from build123d import *

# Parameters (mm, degrees)
F0_W           = 685.8
F0_H           = 1397
F1_DEPTH       = 711.2
F2_W           = 609.6
F2_H           = 508
F2_H_2         = 88.9
F3_DEPTH       = 800.1
F4_W           = 609.6
F4_H           = 88.9
F5_DEPTH       = 596.901
F6_W           = 609.6
F6_H           = 762
F7_DEPTH       = 9.525
F8_W           = 584.2
F8_H           = 736.6
F9_DEPTH       = 50.8
F10_W          = 609.6
F10_H          = 38.1
F11_DEPTH      = 1397.001
F12_W          = 762
F12_H          = 508
F12_W_2        = 1320.8
F12_H_2        = 127
F13_DEPTH      = 685.801
F14_W          = 609.6
F14_H          = 508
F15_DEPTH      = 584.2
F16_W          = 609.6
F16_H          = 520.7
F17_DEPTH      = 9.525
F18_W          = 584.2
F18_H          = 495.3
F19_DEPTH      = 28.575
F21_DEPTH      = 685.801
F22_W          = 558.8
F22_H          = 38.1
F23_DEPTH      = 558.8
F24_W          = 558.7746
F24_H          = 558.8
F24_R          = 228.6
F25_DEPTH      = 50.8
F26_W          = 38.1
F26_H          = 25.4
F27_DEPTH      = 52.5951328439
F28_W          = 38.1
F28_H          = 38.1
F29_DEPTH      = 127
F29_DEPTH_BACK = 88.9
F30_W          = 609.6
F30_H          = 508
F31_DEPTH      = 12.7
F32_W          = 609.6
F32_H          = 762
F33_DEPTH      = 165.101
F34_W          = 38.1
F34_H          = 38.1
F35_DEPTH      = 762


# Not quite as in the source:
# - a length typed as a fraction of an inch, garbled in the dataset ("3 / 203.2 mm" for 3/8 in), is restored


with BuildPart() as f1:
    # F0 (on Top) → F1 (new body)
    with BuildSketch(Plane.XY):
        Rectangle(F0_W, F0_H)
    extrude(amount=F1_DEPTH)

    # F2 (on face) → F3 (cut)
    with BuildSketch(Plane.XZ.offset(698.5)):
        with Locations((0, 419.1)):
            Rectangle(F2_W, F2_H)
        with Locations((0, 82.55)):
            Rectangle(F2_W, F2_H_2)
    extrude(amount=-F3_DEPTH, mode=Mode.SUBTRACT)

    # F4 (on face) → F5 (cut, through all)
    with BuildSketch(Plane.XZ.offset(-101.6)):
        with Locations((0, 82.55)):
            Rectangle(F4_W, F4_H)
    extrude(amount=-F5_DEPTH, mode=Mode.SUBTRACT)

    # F6 (on face) → F7 (cut)
    with BuildSketch(Plane.XY.offset(711.2)):
        with Locations((0, -279.4)):
            Rectangle(F6_W, F6_H)
    extrude(amount=-F7_DEPTH, mode=Mode.SUBTRACT)

    # F8 (on face) → F9 (cut)
    with BuildSketch(Plane.XY.offset(701.675)):
        with Locations((0, -279.4)):
            Rectangle(F8_W, F8_H)
    extrude(amount=-F9_DEPTH, mode=Mode.SUBTRACT)

    # F10 (on face) → F11 (cut, through all)
    with BuildSketch(Plane.XZ.offset(698.5)):
        with Locations((0, 19.05)):
            Rectangle(F10_W, F10_H)
    extrude(amount=-F11_DEPTH, mode=Mode.SUBTRACT)

    # F12 (on face) → F13 (cut, through all)
    with BuildSketch(Plane(origin=(-342.9, 0, 0), x_dir=(0, -1, 0), z_dir=(-1, 0, 0))):
        with Locations((279.4, 419.1)):
            Rectangle(F12_W, F12_H)
        with Locations((0, 63.5)):
            Rectangle(F12_W_2, F12_H_2)
    extrude(amount=-F13_DEPTH, mode=Mode.SUBTRACT)

    # F14 (on face) → F15 (cut)
    with BuildSketch(Plane(origin=(0, 698.5, 0), x_dir=(-1, 0, 0), z_dir=(0, 1, 0))):
        with Locations((0, 419.1)):
            Rectangle(F14_W, F14_H)
    extrude(amount=-F15_DEPTH, mode=Mode.SUBTRACT)

    # F16 (on face) → F17 (cut)
    with BuildSketch(Plane.XY.offset(711.2)):
        with Locations((0, 400.05)):
            Rectangle(F16_W, F16_H)
    extrude(amount=-F17_DEPTH, mode=Mode.SUBTRACT)

    # F18 (on face) → F19 (cut, through all)
    with BuildSketch(Plane.XY.offset(701.675)):
        with Locations((0, 400.05)):
            Rectangle(F18_W, F18_H)
    extrude(amount=-F19_DEPTH, mode=Mode.SUBTRACT)

    # F20 (on face) → F21 (cut, through all)
    with BuildSketch(Plane.YZ.offset(342.9)):
        Polygon((660.4, 673.1), (647.7, 673.1), (152.4, 673.1), (139.7, 673.1), (139.7, 165.1), (660.4, 165.1), align=None)
    extrude(amount=-F21_DEPTH, mode=Mode.SUBTRACT)

    # F22 (on face) → F23 (join)
    with BuildSketch(Plane.YZ.offset(342.9)):
        with Locations((381, 146.05)):
            Rectangle(F22_W, F22_H)
    extrude(amount=F23_DEPTH)

    # F24 (on face) → F25 (join)
    with BuildSketch(Plane.XY.offset(165.1)):
        with Locations((622.3127, 381)):
            Rectangle(F24_W, F24_H)
        with Locations((622.3, 381)):
            Circle(F24_R, mode=Mode.SUBTRACT)
    extrude(amount=F25_DEPTH)

    # F26 (on face) → F27 (cut, up to face)
    with BuildSketch(Plane.XZ.offset(-101.6)):
        with Locations((622.3, 203.2)):
            Rectangle(F26_W, F26_H)
    extrude(amount=-F27_DEPTH, mode=Mode.SUBTRACT)

    # F28 (on face) → F29 (join, two sides)
    with BuildSketch(Plane(origin=(0, 0, 127), x_dir=(1, 0, 0), z_dir=(0, 0, -1))) as f29_sk:
        with Locations((882.65, -82.55)):
            Rectangle(F28_W, F28_H)
        with Locations((882.65, -679.45)):
            Rectangle(F28_W, F28_H)
        with Locations((361.9619884968, -82.55)):
            Rectangle(F28_W, F28_H)
    extrude(amount=F29_DEPTH)
    extrude(f29_sk.sketch, amount=-F29_DEPTH_BACK)

    # F30 (on face) → F31 (cut, through all)
    with BuildSketch(Plane(origin=(0, 114.3, 0), x_dir=(-1, 0, 0), z_dir=(0, 1, 0))):
        with Locations((0, 419.1)):
            Rectangle(F30_W, F30_H)
    extrude(amount=-F31_DEPTH, mode=Mode.SUBTRACT)

    # F32 (on face) → F33 (cut, through all)
    with BuildSketch(Plane.XY.offset(165.1)):
        with Locations((0, -279.4)):
            Rectangle(F32_W, F32_H)
    extrude(amount=-F33_DEPTH, mode=Mode.SUBTRACT)

    # F34 (on face) → F35 (join, through all)
    with BuildSketch(Plane.XZ.offset(-101.6)):
        with Locations((107.95, 146.05)):
            Rectangle(F34_W, F34_H)
        with Locations((-107.95, 146.05)):
            Rectangle(F34_W, F34_H)
    extrude(amount=F35_DEPTH)


solid = f1.part
Design review of the part built by this model. Coordinates are the model's own, in mm. A direction names the side the tool comes from. Give positions to 0.01 mm unless a question says otherwise; leave off trailing zeros. Write each loop counter-clockwise with the first axis right and the second up, starting at its lowest first coordinate (ties: lowest second). Pieces come first, ordered by that corner, then holes. Notation, with made-up numbers: M 75.5,44 L 89.5,44 A17 cw 89.5,58 Z; hole C 24.25,15.5 d9. An arc over 180 degrees is marked long. Return JSON: item names as keys, results as strings. Group by question number.
Item 1: Clearance check with flat-ended pins moving along their axes: pin 1 Ø8 at (x, y) = (128, -185) entering from +Z; pin 2 Ø11.5 at (x, y) = (628.5, 123.5) entering from +Z; pin 3 Ø2 at (x, y) = (454, 535) entering from +Z. State where each tip first meets the part, or that it passes through.
Item 2: Wall thickness on line 1 along X through (y, z) = (381, 197); line 2 along Y through (x, z) = (321, 254); line 3 along Y through (x, z) = (622.3, 183): over which ranges is each line inside the solid? List them lowest first.
Item 3: Take a section at A-A (x = 202). Give the boundary of the cut face in (y, z) (3 decimals), plus the area to 3 significant figures.
Item 4: Tool access review of faces 3 (the cylindrical face through (727.8, 178.2, 190.1)), 4 (the flat face through (-304.8, 121, 416)), 5 (the flat face through (-304.8, -680, 63)), 6 (the flat face through (882, 660.4, 64)), 7 (the flat face through (2, 107, 673.1)): name each direction out of +Z, -Z, +X, -X, +Y, -Y from which nothing blocks a thin tool from reaching the whole face with its end or side.
Item 5: The part is to be moulded in two halves that separate along X. For faces 1 (the flat face through (-217, -660.4, 146)), 2 (the flat face through (-27, 107, 711.2)), say which applies: pulls with the +X half, pulls with the -X half, needs draft (parallel to the pull), parting line crosses it, or undercut.
Item 6: Take a section at B-B (y = -530). Give the boundary of the cut face in (x, z) (3 decimals), plus the area to 3 significant figures.
Item 7: Take a section at D-D (y = 381). Give the boundary of the cut face in (x, z) (3 decimals), plus the area to 3 significant figures.
Item 8: Take a section at C-C (z = 481). Give the boundary of the cut face in (x, y).
Return value:
{
 "1": {"pin 1": "stops at z = 165.1", "pin 2": "stops at z = 190.5", "pin 3": "stops at z = 215.9"},
 "2": {"line 1": "x = 342.93 to 393.7, 850.9 to 901.7", "line 2": "y = -698.5 to -660.4, 101.6 to 139.7, 660.4 to 698.5", "line 3": "y = 101.6 to 152.4, 609.6 to 660.4"},
 "3": {"outline": "M -698.5,127 L -660.4,127 L -660.4,165.1 L -698.5,165.1 Z; M -698.5,673.1 L -647.7,673.1 L -647.7,701.675 L -660.4,701.675 L -660.4,711.2 L -698.5,711.2 Z; M 88.9,673.1 L 152.4,673.1 L 152.4,701.675 L 139.7,701.675 L 139.7,711.2 L 101.6,711.2 L 101.6,701.675 L 88.9,701.675 Z; M 101.6,127 L 698.5,127 L 698.5,165.1 L 101.6,165.1 Z; M 647.7,673.1 L 698.5,673.1 L 698.5,711.2 L 660.4,711.2 L 660.4,701.675 L 647.7,701.675 Z", "area": "30,000 mm2"},
 "4": {"face 3": "+Z", "face 4": "+Y, -Y", "face 5": "-Z, +Y, -Y", "face 6": "-Z, +X, -X", "face 7": "none"},
 "5": {"face 1": "undercut", "face 2": "needs draft"},
 "6": {"outline": "M -342.9,127 L -304.8,127 L -304.8,165.1 L -342.9,165.1 Z; M -342.9,673.1 L -292.1,673.1 L -292.1,701.675 L -304.8,701.675 L -304.8,711.2 L -342.9,711.2 Z; M -127,127 L -88.9,127 L -88.9,165.1 L -127,165.1 Z; M 88.9,127 L 127,127 L 127,165.1 L 88.9,165.1 Z; M 292.1,673.1 L 342.9,673.1 L 342.9,711.2 L 304.8,711.2 L 304.8,701.675 L 292.1,701.675 Z; M 304.8,127 L 342.9,127 L 342.9,165.1 L 304.8,165.1 Z", "area": "9,440 mm2"},
 "7": {"outline": "M -342.9,127 L 901.7,127 L 901.7,215.9 L 850.9,215.9 L 850.9,165.1 L 393.7,165.1 L 393.7,215.9 L 342.925,215.9 L 342.925,165.1 L -342.9,165.1 Z; M -342.9,673.1 L -292.1,673.1 L -292.1,701.675 L -304.8,701.675 L -304.8,711.2 L -342.9,711.2 Z; M 292.1,673.1 L 342.9,673.1 L 342.9,711.2 L 304.8,711.2 L 304.8,701.675 L 292.1,701.675 Z", "area": "56,200 mm2"},
 "8": {"outline": "M -342.9,-698.5 L -304.8,-698.5 L -304.8,-660.4 L -342.9,-660.4 Z; M -342.9,101.6 L -304.8,101.6 L -304.8,139.7 L -342.9,139.7 Z; M -342.9,660.4 L -304.8,660.4 L -304.8,698.5 L -342.9,698.5 Z; M 304.8,-698.5 L 342.9,-698.5 L 342.9,-660.4 L 304.8,-660.4 Z; M 304.8,101.6 L 342.9,101.6 L 342.9,139.7 L 304.8,139.7 Z; M 304.8,660.4 L 342.9,660.4 L 342.9,698.5 L 304.8,698.5 Z"}
}
